from build123d import *

# Parameters (mm, degrees)
SKETCH001_W            = 200
SKETCH001_H            = 260
PAD_DEPTH              = 1.5
SKETCH002_W            = 5
SKETCH002_H            = 260
PAD001_DEPTH           = 43.5
PAD004_DEPTH           = 195
SKETCH003_R            = 2.5
PAD002_DEPTH           = 1.5
LINEARPATTERN_COUNT    = 5
LINEARPATTERN_PITCH    = 60
SKETCH004_R            = 1.5
PAD003_DEPTH           = 45
SKETCH006_R            = 2.5
PAD005_DEPTH           = 1.5
LINEARPATTERN001_COUNT = 4
LINEARPATTERN001_PITCH = 60
FILLET002_R            = 1


with BuildPart() as part:
    # Sketch001 (on XY_Plane of Origin) → Pad (new body)
    with BuildSketch(Plane.XY):
        with Locations((100, 130)):
            Rectangle(SKETCH001_W, SKETCH001_H)
    extrude(amount=PAD_DEPTH)

    # Sketch002 (on Face6 of Pad) → Pad001 (join)
    with BuildSketch(Plane.XY.offset(1.5)):
        with Locations((2.5, 130)):
            Rectangle(SKETCH002_W, SKETCH002_H)
    extrude(amount=PAD001_DEPTH)

    # Sketch005 (on Face4 of Pad001) → Pad004 (join)
    with BuildSketch(Plane.YZ.offset(5)):
        Polygon((0, 1.5), (0, 4.5), (2, 4.5), (5, 1.5), align=None)
    extrude(amount=PAD004_DEPTH)

    # Sketch003 (on XY_Plane of Origin) → Pad002 (join)
    with BuildSketch(Plane.XY):
        with Locations((202, 10)):
            Circle(SKETCH003_R)
    pad002 = extrude(amount=PAD002_DEPTH)

    # LinearPattern: Pad002 ×5
    with Locations(*[(0, i * LINEARPATTERN_PITCH, 0) for i in range(1, LINEARPATTERN_COUNT)]):
        add(pad002)

    # Sketch004 (on XY_Plane of Origin) → Pad003 (join)
    with BuildSketch(Plane.XY):
        with Locations((2.5, 261)):
            Circle(SKETCH004_R)
    extrude(amount=PAD003_DEPTH)

    # Sketch006 (on XY_Plane of Origin) → Pad005 (join)
    with BuildSketch(Plane.XY):
        with Locations((190, 262)):
            Circle(SKETCH006_R)
    pad005 = extrude(amount=PAD005_DEPTH)

    # LinearPattern001: Pad005 ×4
    with Locations(*[(-i * LINEARPATTERN001_PITCH, 0, 0) for i in range(1, LINEARPATTERN001_COUNT)]):
        add(pad005)

    # Fillet002
    fillet002_edges = [part.edges().sort_by_distance(p)[0] for p in [
        (0, 130, 45),
        (5, 130, 45),
        (2.5, 0, 45),
        (0, 0, 22.5),
        (5, 0, 24.75),
    ]]
    fillet(fillet002_edges, radius=FILLET002_R)


solid = part.part
Check sheet for the modelled part. Datum: model origin and axes. Units: mm. A direction names the side the tool comes from. Round coordinates to 2 decimals unless told otherwise and drop trailing zeros. Order: outer loops, then holes, each group sorted by start corner. A loop starts at its lowest first (then second) coordinate and runs counter-clockwise, first axis right, second up.
Q1. Cross-section at C-C, the plane y = 43. Enter the section's corners in (x, z).
Filled sheet:
outline: (0, 0) - (200, 0) - (200, 1.5) - (5, 1.5) - (5, 44) arc R1 ccw to (4, 45) - (1, 45) arc R1 ccw to (0, 44) - close
Q2. Cross-section at B-B, the plane x = 143. Enter the section's corners in (y, z).
Filled sheet:
outline: (0, 0) - (260, 0) - (260, 1.5) - (5, 1.5) - (2, 4.5) - (0, 4.5) - close
Q3. Cross-section at A-A, the plane z = 37.5. Enter the section's corners in (x, y), plus the area to 3 significant figures.
Filled sheet:
outline: (0, 1) arc R1 ccw to (1, 0) - (4, 0) arc R1 ccw to (5, 1) - (5, 260) - (3.62, 260) arc R1.5 ccw (long way) to (1.38, 260) - (0, 260) - close
area: 1,310 mm2
Q4. Scan lines: L1, parallel to Z at x = 183, y = 120; L2, parallel to X at y = 251, z = 25. Record each from-to range of solid material in increasing order.
Filled sheet:
L1: z = 0 to 1.5
L2: x = 0 to 5
Q5. Set-up check for faces 1 (the face through (0, 129, 22)), 2 (the face through (103, 137, 1.5)): record each of +Z, -Z, +X, -X, +Y, -Y from which the full face is reachable in a straight line by a thin tool's end or side.
Filled sheet:
face 1: +Z, -Z, -X, +Y, -Y
face 2: +Z, +X, +Y
Q6. Depth check by flat-ended pin: P1, Ø0.8, axis at y = 40.5, z = 1, coming from the +X side; P2, Ø1.2, axis at x = 32.5, z = 0.5, coming from the +Y side; P3, Ø10, axis at y = 89.5, z = 8, coming from the +X side; P4, Ø10, axis at x = 79.5, z = 6.5, coming from the -Y side. Enter the tip coordinate at first touch or a pass-through.
Filled sheet:
P1: stops at x = 200
P2: stops at y = 260
P3: stops at x = 5
P4: stops at y = 0
